Autodesk Inventor part; units mm, degrees
sketch "Boceto1" plane through (0, 0, 0) normal (0, 0, 1) x (1, 0, 0)
  line L0 (-2.5, -10.4) -> (2.5, -10.4)
  line L1 (2.5, -10.4) -> (2.5, 10.4)
  line L2 (2.5, 10.4) -> (-2.5, 10.4)
  line L3 (-2.5, 5.4) -> (-2.5, -5.4)
  line L4 (-2.5, -10.4) -> (2.5, 10.4) construction
  line L5 (2.5, -10.4) -> (-2.5, 10.4) construction
  line L6 (-2.5, 10.4) -> (-22.5, 10.4)
  line L7 (-22.5, 10.4) -> (-22.5, 5.4)
  line L8 (-22.5, 5.4) -> (-2.5, 5.4)
  line L9 (-27.5, 0) -> (7.5, 0)
  line L10 (-2.5, -10.4) -> (-22.5, -10.4)
  line L11 (-22.5, -10.4) -> (-22.5, -5.4)
  line L12 (-22.5, -5.4) -> (-2.5, -5.4)
  point P0 (0, 0)
  dimension "d4" = 25
  dimension "d5" = 20
  dimension "d6" = 10.8
  dimension "d8" = 20.8
extrude "Extrusión1" add sketch "Boceto1" along normal blind 15
sketch "Boceto2" plane through (-22.5, -10.4, 0) normal (0, -1, 0) x (1, 0, 0)
  line L0 (0, 0) -> (0, 15)
  line L1 (0, 15) -> (25, 15)
  line L2 (2, 12.5) -> (6, 12.5)
  line L3 (6, 2.5) -> (2, 2.5)
  line L4 (2, 12.5) -> (6, 2.5) construction
  line L5 (6, 12.5) -> (2, 2.5) construction
  line L6 (4.8542, 9.6355) -> (6, 12.5)
  line L7 (3.1458, 9.6355) -> (2, 12.5)
  line L8 (3.1458, 5.3645) -> (2, 2.5)
  line L9 (4.8542, 5.3645) -> (6, 2.5)
  arc A0 (4.8542, 5.3645) -> (4.8542, 9.6355) centre (4, 7.5) ccw
  arc A1 (3.1458, 9.6355) -> (3.1458, 5.3645) centre (4, 7.5) ccw
  point P0 (22.5, 0)
  point P1 (0, 7.5)
  dimension "d11" = 4
  dimension "d13" = 7.5
  dimension "d25" = 2.3
  dimension "d26" = 2.3
extrude "Extrusión2" cut sketch "Boceto2" against normal blind 2.5
sketch "Boceto3" plane through (-22.5, -7.9, 0) normal (0, -1, 0) x (1, 0, 0)
  arc A0 (4.8542, 5.3645) -> (4.8542, 9.6355) centre (4, 7.5) ccw
  arc A1 (3.1458, 9.6355) -> (3.1458, 5.3645) centre (4, 7.5) ccw
  circle A2 centre (4, 7.5) radius 2.3
  point P0 (22.5, 0)
  point P1 (3.1458, 5.3645)
  point P2 (4.8542, 5.3645)
  point P3 (4.8542, 9.6355)
  point P4 (3.1458, 9.6355)
  dimension "d27" = 4.6
extrude "Extrusión3" cut sketch "Boceto3" against normal blind 2.5
sketch "Boceto4" plane through (-22.5, 10.4, 0) normal (0, 1, 0) x (1, 0, 0)
  circle A0 centre (4, -7.5) radius 2.3 construction
  line L0 (6.3, -8.8279) -> (4, -10.1558)
  line L1 (4, -10.1558) -> (1.7, -8.8279)
  line L2 (1.7, -8.8279) -> (1.7, -6.1721)
  line L3 (1.7, -6.1721) -> (4, -4.8442)
  line L4 (4, -4.8442) -> (6.3, -6.1721)
  line L5 (6.3, -6.1721) -> (6.3, -8.8279)
  point P0 (22.5, 0)
  point P1 (6.3, -7.5)
extrude "Extrusión4" cut sketch "Boceto4" against normal blind 2.5
sketch "Boceto5" plane through (-22.5, 7.9, 0) normal (0, 1, 0) x (1, 0, 0)
  arc A0 (4.8542, -9.6355) -> (4.8542, -5.3645) centre (4, -7.5) ccw
  circle A1 centre (4, -7.5) radius 1.75
  point P0 (22.5, 0)
  point P1 (3.1458, -5.3645)
  point P2 (3.1458, -9.6355)
  dimension "d22" = 3.5
extrude "Extrusión5" cut sketch "Boceto5" against normal blind 2.5
properties part number "PruebaCParaBuje_3DPrint"
Here's how the part is built. I have some questions about the finished solid (model axes, mm). A direction names the side the tool comes from. Give positions to 0.01 mm unless a question says otherwise; leave off trailing zeros. Write each loop counter-clockwise with the first axis right and the second up, starting at its lowest first coordinate (ties: lowest second). Pieces come first, ordered by that corner, then holes. Notation, with made-up numbers: (-34.5, 22) -> (-27.5, 22) arc R32 cw to (-27.5, 48) -> close; hole circle Ø5 at (3.5, 33). An arc over 180 degrees is marked (long way). Use one line per item in the form item = value.
1) We'd pull the mould along X, two halves only. Please class faces 1 (the face through (-2.5, 0, 7)), 2 (the face through (2.5, 0, 7)), 3 (the face through (-20.8, 9, 8)), 4 (the face through (-13, 5.4, 7)): +X half, -X half, draft (parallel to the pull), parting line (faces both ways), or undercut.
Verdict:
face_1 = -X half
face_2 = +X half
face_3 = undercut
face_4 = draft
2) I'm going to push flat-ended pins straight in: pin 1 (2 mm diameter, centred on x = -18.5, z = 7.5, fed in from -Y) (3 decimals); pin 2 (3 mm diameter, centred on y = -0.5, z = 5, fed in from -X); pin 3 (1.4 mm diameter, centred on x = -18, z = 3.5, fed in from -Y). Where does each tip first touch, or does it pass through?
Verdict:
pin_1 = through
pin_2 = -2.5
pin_3 = -7.9
3) Suppose I cut it at A-A (x = -3.75). Please give me the cut outline in (y, z), and give its area (3 significant figures).
Verdict:
outline = (-10.4, 0) -> (-5.4, 0) -> (-5.4, 15) -> (-10.4, 15) -> close; (5.4, 0) -> (10.4, 0) -> (10.4, 15) -> (5.4, 15) -> close
area = 150 mm2
4) If I drill on L1, parallel to Y at x = -19.75, z = 14; L2, parallel to Z at x = -18.5, y = 6; L3, parallel to Y at x = -18.25, z = 12.25, over which ranges is the centre line in solid material (lowest first)? Write a range as [from, to].
Verdict:
L1 = [-10.4, -5.4], [5.4, 10.4]
L2 = [0, 5.75], [9.25, 15]
L3 = [-7.9, -5.4], [5.4, 10.4]
5) Suppose I cut it at C-C (z = 7.5). Please give me the cut outline in (x, y).
Verdict:
outline = (-22.5, -10.4) -> (-20.8, -10.4) -> (-20.8, -5.4) -> (-22.5, -5.4) -> close; (-22.5, 5.4) -> (-20.25, 5.4) -> (-20.25, 7.9) -> (-20.8, 7.9) -> (-20.8, 10.4) -> (-22.5, 10.4) -> close; (-16.75, 5.4) -> (-2.5, 5.4) -> (-2.5, -5.4) -> (-16.2, -5.4) -> (-16.2, -10.4) -> (2.5, -10.4) -> (2.5, 10.4) -> (-16.2, 10.4) -> (-16.2, 7.9) -> (-16.75, 7.9) -> close
6) On a 3-axis mill with a long thin cutter (end or side, diameter ignored), from which of +Z, -Z, +X, -X, +Y, -Y can I reach the whole of each face in a straight line? I mean faces 5 (the face through (-2, 0, 0)), 6 (the face through (-10, 10.4, 7)), 7 (the face through (-19.634, 9.168, 9.501)), 8 (the face through (-19.9, -9.2, 11)), 9 (the face through (-13, -5.4, 7)). Say none if no direction works.
Verdict:
face_5 = -Z, +X, -X, +Y, -Y
face_6 = +Z, -Z, +X, -X, +Y
face_7 = +Y
face_8 = -Y
face_9 = +Z, -Z, -X
7) Suppose I cut it at D-D (z = 13.5). Please give me the cut outline in (x, y), and give its area (3 significant figures).
Verdict:
outline = (-22.5, -10.4) -> (2.5, -10.4) -> (2.5, 10.4) -> (-22.5, 10.4) -> (-22.5, 5.4) -> (-2.5, 5.4) -> (-2.5, -5.4) -> (-22.5, -5.4) -> close
area = 304 mm2
8) Suppose I cut it at B-B (y = -7.5). Please give me the cut outline in (x, z), and give its area (3 significant figures).
Verdict:
outline = (-22.5, 0) -> (2.5, 0) -> (2.5, 15) -> (-22.5, 15) -> close; hole (-19.35, 9.64) arc R2.3 ccw (long way) to (-17.65, 9.64) arc R2.3 ccw to start
area = 358 mm2
